Build history of the part. All positions in model axes, mm. A direction names the side the tool comes from. Coordinates: 2 decimals unless noted, no trailing zeros. Write each loop counter-clockwise with the first axis right and the second up, starting at its lowest first coordinate (ties: lowest second). Pieces come first, ordered by that corner, then holes. Notation, with made-up numbers: (56, 58) -> (115, 58) arc R10 cw to (115, 72) -> close; hole circle Ø4 at (-26.75, 53.25). An arc over 180 degrees is marked (long way). Write each question's results on one line, items separated by ' | '. Start each with the question number.
Q1. Saw through at C-C on x = 23.5. Give the cut face in (y, z), and give its area (3 significant figures).
Q2. Saw through at A-A on z = 1.05. Give the cut face in (x, y), and give its area (3 significant figures).
Q3. Drill centre lines: line 1 (Y direction, x = 0, z = 0.55); line 2 (Y direction, x = 36, z = 0.2); line 3 (Y direction, x = 3.5, z = 0.2). Where is each one in solid material? Low to high.
Q4. Tool access for faces 1 (the face through (18, 0, 0)), 2 (the face through (35, -2.6, 1)): list every direction of +Z, -Z, +X, -X, +Y, -Y with a clear straight run to the whole face (end or side of a thin tool).
Q5. Saw through at D-D on y = 3.75. Give the cut face in (x, z), and give its area (3 significant figures).
Q6. Two-plate mould, pull along Y, no slides. Class faces 3 (the face through (0, 1, 1)), 4 (the face through (16.584, 3.785, 0.986)), 5 (the face through (16.584, -3.785, 0.986)): released by +Y, released by -Y, zero draft, split by the parting line, or undercut.
Q7. Drop flat-ended pins along their axis: pin 1 Ø1 at (y, z) = (-3.5, 1.5) entering from +X; pin 2 Ø1 at (x, z) = (25.5, 0.5) entering from +Y. Give the stop position or say it passes through.
Q8. Saw through at B-B on y = 0. Give the cut face in (x, z).
Autodesk Inventor part; units mm, degrees
ref_plane "YZ Plane" through (0, 0, 0) normal (1, 0, 0) x (0, 1, 0)
ref_plane "XZ Plane" through (0, 0, 0) normal (0, 1, 0) x (-1, 0, 0)
ref_plane "XY Plane" through (0, 0, 0) normal (0, 0, 1) x (1, 0, 0)
sketch "Sketch1" plane through (0, 0, 0) normal (0, 0, 1) x (1, 0, 0)
  circle A0 centre (0, 0) radius 1
  arc A1 (34, 2.6) -> (34, -2.6) centre (34, 0) ccw
  line L0 (34, 2.6) -> (36, 2.6)
  line L1 (34, -2.6) -> (36, -2.6)
  arc A2 (36, -2.6) -> (36, 2.6) centre (36, 0) ccw
  arc A3 (-0.1412, 2.9967) -> (-0.1412, -2.9967) centre (0, 0) ccw
  line L2 (34, 4.6) -> (36, 4.6)
  arc A4 (36, -4.6) -> (36, 4.6) centre (36, 0) ccw
  line L3 (36, -4.6) -> (34, -4.6)
  line L4 (-0.1412, 2.9967) -> (33.7835, 4.5949)
  line L5 (12.7162, 0) -> (28.1806, 0)
  line L6 (-0.1412, -2.9967) -> (33.7835, -4.5949)
  arc A5 (34, 4.6) -> (33.7835, 4.5949) centre (34, 0) ccw
  arc A6 (33.7835, -4.5949) -> (34, -4.6) centre (34, 0) ccw
  dimension "d0" = 2
  dimension "d1" = 5.2
  dimension "d2" = 34
  dimension "d3" = 2
  dimension "d4" = 2
extrude "Extrusion1" add sketch "Sketch1" along normal blind 2
properties part number "rotasyonpini"
Returned:
1) outline: (-4.11, 0) -> (4.11, 0) -> (4.11, 2) -> (-4.11, 2) -> close | area: 16.4 mm2
2) outline: (-0.14, -3) -> (33.78, -4.59) arc R4.6 ccw to (34, -4.6) -> (36, -4.6) arc R4.6 ccw to (36, 4.6) -> (34, 4.6) arc R4.6 ccw to (33.78, 4.59) -> (-0.14, 3) arc R3 ccw to start; hole circle Ø2 at (0, 0); hole (34, -2.6) -> (36, -2.6) arc R2.6 ccw to (36, 2.6) -> (34, 2.6) arc R2.6 ccw to start | area: 290 mm2
3) line 1: y = -3 to -1, 1 to 3 | line 2: y = -4.6 to -2.6, 2.6 to 4.6 | line 3: y = -3.17 to 3.17
4) face 1: -Z, +X, -X, +Y, -Y | face 2: +Z, -Z
5) outline: (15.85, 0) -> (38.66, 0) -> (38.66, 2) -> (15.85, 2) -> close | area: 45.6 mm2
6) face 3: undercut | face 4: released by +Y | face 5: released by -Y
7) pin 1: stops at x = 39.49 | pin 2: stops at y = 4.23
8) outline: (-3, 0) -> (-1, 0) -> (-1, 2) -> (-3, 2) -> close; (1, 0) -> (31.4, 0) -> (31.4, 2) -> (1, 2) -> close; (38.6, 0) -> (40.6, 0) -> (40.6, 2) -> (38.6, 2) -> close
